```python
from build123d import *

# Parameters (mm, degrees)
SKETCH1_R           = 20.0025
BOSS_EXTRUDE1_DEPTH = 5.08
SKETCH2_W           = 1.8
SKETCH2_H           = 15.24
BOSS_EXTRUDE2_DEPTH = 1.8
FILLET1_R           = 0.9


with BuildPart() as part:
    # Sketch1 → Boss-Extrude1 (new body)
    with BuildSketch(Plane(origin=(0, 0, 0), x_dir=(1, 0, 0), z_dir=(0, 1, 0))):
        with Locations(Location((0, 0, 0), (0, 0, 270))):
            Circle(SKETCH1_R)
    extrude(amount=BOSS_EXTRUDE1_DEPTH)

    # Sketch2 → Boss-Extrude2 (add)
    with BuildSketch(Plane.XZ):
        with Locations((-5.45, 20.32)):
            Rectangle(SKETCH2_W, SKETCH2_H)
        with Locations((5.45, 20.32)):
            Rectangle(SKETCH2_W, SKETCH2_H)
    extrude(amount=-BOSS_EXTRUDE2_DEPTH)

    # Fillet1
    fillet1_edges = [part.edges().sort_by_distance(p)[0] for p in [
        (6.35, 1.8, 23.453900915),
        (6.35, 0, 23.453900915),
        (4.55, 1.8, 23.70906446),
        (4.55, 0, 23.70906446),
        (-6.35, 1.8, 23.453900915),
        (-4.55, 1.8, 23.70906446),
        (-6.35, 0, 23.453900915),
        (-4.55, 0, 23.70906446),
    ]]
    fillet(fillet1_edges, radius=FILLET1_R - 0.0001)  # a hair under: the kernel refuses the full size


solid = part.part
```
Can you work these out from the model? Positions are in its coordinate system, mm. Coordinates: 2 decimals unless noted, no trailing zeros. Loops run counter-clockwise (first coordinate to the right, second up) from the corner with the lowest first, then second, coordinate; pieces in that order, holes last.
1) For pin 1 (1 mm diameter, centred on x = -12, y = 1, fed in from -Z); pin 2 (2 mm diameter, centred on x = 14, y = 1.5, fed in from -Z); pin 3 (3 mm diameter, centred on x = 15, y = 2, fed in from -Z), each with a flat end and sliding along its axis, tell me the tip position at first contact or that it passes through.
2) Imagine slicing it at A-A on y = 4.15. List the corners of the cut face in (x, z) for me (1 decimal).
3) Imagine slicing it at B-B on x = -12.5. List the corners of the cut face in (y, z) for me, plus the area to 3 significant figures.
4) Imagine slicing it at C-C on z = 3.5. List the corners of the cut face in (x, y) for me.
5) I need wall thicknesses on probe 1 along X at (y, z) = (1.4, 26); probe 2 along X at (y, z) = (1.7, -15); probe 3 along Z at (x, y) = (10.5, 4.8). Which ranges of each line are inside material? Lowest first, please.
Completed:
1. pin 1: stops at z = -16.37
1. pin 2: stops at z = -15.2
1. pin 3: stops at z = -14.76
2. outline: circle Ø40 at (0, 0)
3. outline: (0, -15.62) - (5.08, -15.62) - (5.08, 15.62) - (0, 15.62) - close
3. area: 159 mm2
4. outline: (-19.69, 0) - (19.69, 0) - (19.69, 5.08) - (-19.69, 5.08) - close
5. probe 1: x = -6.2 to -4.7, 4.7 to 6.2
5. probe 2: x = -13.23 to 13.23
5. probe 3: z = -17.02 to 17.02
